from build123d import *

# Parameters (mm, degrees)
SKETCH_1_W          = 80
SKETCH_1_H          = 20
SKETCH_1_R          = 1
EXTRUDE_1_DEPTH     = 1.6
CUT_EXTRUDE_1_DEPTH = 0.1
CUT_EXTRUDE_START   = -0.1
CUT_EXTRUDE_2_DEPTH = 0.1


with BuildPart() as part:
    # Эскиз1 → Бобышка-Вытянуть1 (new body)
    with BuildSketch(Plane.XY):
        Rectangle(SKETCH_1_W, SKETCH_1_H)
        with Locations((-37.5, 7.5)):
            Circle(SKETCH_1_R, mode=Mode.SUBTRACT)
        with Locations((-37.5, -7.5)):
            Circle(SKETCH_1_R, mode=Mode.SUBTRACT)
        with Locations((37.5, -7.5)):
            Circle(SKETCH_1_R, mode=Mode.SUBTRACT)
        with Locations((37.5, 7.5)):
            Circle(SKETCH_1_R, mode=Mode.SUBTRACT)
    extrude(amount=EXTRUDE_1_DEPTH)

    # Эскиз2 → Вырез-Вытянуть1 (cut)
    with BuildSketch(Plane.XY.offset(1.6)):
        with BuildLine():
            Line((-38, -2.75), (-35.5, -2.75))
            ThreePointArc((-35.5, -2.75), (-34.5, -3.75), (-35.5, -4.75))
            Line((-35.5, -4.75), (-38, -4.75))
            ThreePointArc((-38, -4.75), (-39, -3.75), (-38, -2.75))
        make_face()
        with BuildLine():
            Line((-38, -0.25), (-35.5, -0.25))
            ThreePointArc((-35.5, -0.25), (-34.5, -1.25), (-35.5, -2.25))
            Line((-35.5, -2.25), (-38, -2.25))
            ThreePointArc((-38, -2.25), (-39, -1.25), (-38, -0.25))
        make_face()
        with BuildLine():
            Line((-38, 2.25), (-35.5, 2.25))
            ThreePointArc((-35.5, 2.25), (-34.5, 1.25), (-35.5, 0.25))
            Line((-35.5, 0.25), (-38, 0.25))
            ThreePointArc((-38, 0.25), (-39, 1.25), (-38, 2.25))
        make_face()
        with BuildLine():
            Line((38, -2.75), (35.5, -2.75))
            ThreePointArc((35.5, -2.75), (34.5, -3.75), (35.5, -4.75))
            Line((35.5, -4.75), (38, -4.75))
            ThreePointArc((38, -4.75), (39, -3.75), (38, -2.75))
        make_face()
        with BuildLine():
            Line((-38, 4.75), (-35.5, 4.75))
            ThreePointArc((-35.5, 4.75), (-34.5, 3.75), (-35.5, 2.75))
            Line((-35.5, 2.75), (-38, 2.75))
            ThreePointArc((-38, 2.75), (-39, 3.75), (-38, 4.75))
        make_face()
        with BuildLine():
            Line((38, -0.25), (35.5, -0.25))
            ThreePointArc((35.5, -0.25), (34.5, -1.25), (35.5, -2.25))
            Line((35.5, -2.25), (38, -2.25))
            ThreePointArc((38, -2.25), (39, -1.25), (38, -0.25))
        make_face()
        with BuildLine():
            Line((38, 2.25), (35.5, 2.25))
            ThreePointArc((35.5, 2.25), (34.5, 1.25), (35.5, 0.25))
            Line((35.5, 0.25), (38, 0.25))
            ThreePointArc((38, 0.25), (39, 1.25), (38, 2.25))
        make_face()
        with BuildLine():
            Line((38, 4.75), (35.5, 4.75))
            ThreePointArc((35.5, 4.75), (34.5, 3.75), (35.5, 2.75))
            Line((35.5, 2.75), (38, 2.75))
            ThreePointArc((38, 2.75), (39, 3.75), (38, 4.75))
        make_face()
    extrude(amount=-CUT_EXTRUDE_1_DEPTH, mode=Mode.SUBTRACT)

    # Эскиз3 → Вырез-Вытянуть2 (cut)
    with BuildSketch(Plane(origin=(0, 0, 0), x_dir=(-1, 0, 0), z_dir=(0, 0, -1)).offset(CUT_EXTRUDE_START)):
        with BuildLine():
            Line((38, -0.25), (35.5, -0.25))
            ThreePointArc((35.5, -0.25), (34.5, -1.25), (35.5, -2.25))
            Line((35.5, -2.25), (38, -2.25))
            ThreePointArc((38, -2.25), (39, -1.25), (38, -0.25))
        make_face()
        with BuildLine():
            Line((38, -2.75), (35.5, -2.75))
            ThreePointArc((35.5, -2.75), (34.5, -3.75), (35.5, -4.75))
            Line((35.5, -4.75), (38, -4.75))
            ThreePointArc((38, -4.75), (39, -3.75), (38, -2.75))
        make_face()
        with BuildLine():
            Line((38, 2.25), (35.5, 2.25))
            ThreePointArc((35.5, 2.25), (34.5, 1.25), (35.5, 0.25))
            Line((35.5, 0.25), (38, 0.25))
            ThreePointArc((38, 0.25), (39, 1.25), (38, 2.25))
        make_face()
        with BuildLine():
            Line((-35.5, -0.25), (-38, -0.25))
            ThreePointArc((-38, -0.25), (-39, -1.25), (-38, -2.25))
            Line((-38, -2.25), (-35.5, -2.25))
            ThreePointArc((-35.5, -2.25), (-34.5, -1.25), (-35.5, -0.25))
        make_face()
        with BuildLine():
            Line((-35.5, -2.75), (-38, -2.75))
            ThreePointArc((-38, -2.75), (-39, -3.75), (-38, -4.75))
            Line((-38, -4.75), (-35.5, -4.75))
            ThreePointArc((-35.5, -4.75), (-34.5, -3.75), (-35.5, -2.75))
        make_face()
        with BuildLine():
            Line((-35.5, 2.25), (-38, 2.25))
            ThreePointArc((-38, 2.25), (-39, 1.25), (-38, 0.25))
            Line((-38, 0.25), (-35.5, 0.25))
            ThreePointArc((-35.5, 0.25), (-34.5, 1.25), (-35.5, 2.25))
        make_face()
        with BuildLine():
            Line((38, 4.75), (35.5, 4.75))
            ThreePointArc((35.5, 4.75), (34.5, 3.75), (35.5, 2.75))
            Line((35.5, 2.75), (38, 2.75))
            ThreePointArc((38, 2.75), (39, 3.75), (38, 4.75))
        make_face()
        with BuildLine():
            Line((-35.5, 4.75), (-38, 4.75))
            ThreePointArc((-38, 4.75), (-39, 3.75), (-38, 2.75))
            Line((-38, 2.75), (-35.5, 2.75))
            ThreePointArc((-35.5, 2.75), (-34.5, 3.75), (-35.5, 4.75))
        make_face()
    extrude(amount=CUT_EXTRUDE_2_DEPTH, mode=Mode.SUBTRACT)


solid = part.part
Geometry: final body of the model. Coordinates: model frame, mm. A direction names the side the tool comes from. Round coordinates to 2 decimals unless told otherwise and drop trailing zeros. Loops run counter-clockwise (first coordinate to the right, second up) from the corner with the lowest first, then second, coordinate; pieces in that order, holes last. Notation, with made-up numbers: (28, -32.5) - (59, -32.5) arc R25 cw to (59, -17.5) - close; hole circle Ø8 at (76, 18). An arc over 180 degrees is marked (long way). Write each question's results on one line, items separated by ' | '. Start each with the question number.
1) Line query: probe 1 along Y at (x, z) = (37.5, 0.6). Output: solid intervals per line, ascending. Write a range as [from, to].
2) Access query for faces 5 (the face through (-37, -1, 0.1)), 6 (the face through (-37, 4, 1.5)), 7 (the face through (-1, 0, 1.6)). Directions: +Z, -Z, +X, -X, +Y, -Y. A direction counts if a zero-diameter tool reaches every point of the face in a straight line with its end or side. Return the directions, or none.
3) Cut plane A-A on y = 7.5. Return loops of the section in (x, z), then the cut area to 3 significant figures.
4) First-contact query: P1, Ø0.6, axis at x = 37.5, y = -3.5, coming from the -Z side; P2, Ø0.6, axis at x = -37.5, y = 4, coming from the +Z side. Flat tips, straight axial feed; report the tip coordinate or a pass-through.
5) Mould query, pull axis Y, two halves, no side actions, for faces 1 (the face through (-1, 10, 1)), 2 (the face through (37, 4, 1.5)), 3 (the face through (-37, -1, 1.5)), 4 (the face through (-40, 0, 1)). Classes: released by +Y, released by -Y, zero draft, split by the parting line, or undercut.
Verdict:
1) probe 1: y = [-10, -8.5], [-6.5, 6.5], [8.5, 10]
2) face 5: -Z | face 6: +Z | face 7: +Z, +X, -X, +Y, -Y
3) outline: (-40, 0) - (-38.5, 0) - (-38.5, 1.6) - (-40, 1.6) - close; (-36.5, 0) - (36.5, 0) - (36.5, 1.6) - (-36.5, 1.6) - close; (38.5, 0) - (40, 0) - (40, 1.6) - (38.5, 1.6) - close | area: 122 mm2
4) P1: stops at z = 0.1 | P2: stops at z = 1.5
5) face 1: released by +Y | face 2: undercut | face 3: undercut | face 4: zero draft
